Autodesk Fusion 360 part; units mm, degrees
sketch "Sketch1" plane through (0, 0, 0) normal (0, 1, 0) x (1, 0, 0)
  line L0 (37.303, -16.4637) -> (7.303, -16.4637)
  line L1 (-2.697, -16.4637) -> (-2.697, -12.4637)
  line L2 (2.303, -12.4637) -> (37.303, -12.4637)
  line L3 (37.303, -12.4637) -> (37.303, -16.4637)
  line L4 (37.303, -18.5137) -> (-5.6588, -18.5137) construction
  line L5 (2.303, -24.5637) -> (37.303, -24.5637)
  line L6 (-2.697, -20.5637) -> (-2.697, -24.5637)
  line L7 (37.303, -20.5637) -> (7.303, -20.5637)
  line L8 (37.303, -24.5637) -> (37.303, -20.5637)
  line L9 (-2.697, -16.4637) -> (-2.697, -20.5637)
  line L10 (7.303, -16.4637) -> (7.303, -20.5637)
  line L11 (2.303, -12.4637) -> (2.303, -2.4637)
  line L12 (2.303, -2.4637) -> (-2.697, -2.4637)
  line L13 (-2.697, -2.4637) -> (-2.697, -12.4637)
  line L14 (-2.697, -34.5637) -> (-2.697, -24.5637)
  line L15 (2.303, -34.5637) -> (-2.697, -34.5637)
  line L16 (2.303, -24.5637) -> (2.303, -34.5637)
  dimension "d4" = 4
  dimension "d5" = 10
  dimension "d6" = 5
  dimension "d7" = 10
extrude "Extrude1" add sketch "Sketch1" along normal blind 60
sketch "Sketch2" plane through (-2.697, 0, 0) normal (-1, 0, 0) x (0, -1, 0)
  line L0 (0, 2.4637) -> (0, 34.5637)
  line L1 (0, 34.5637) -> (-60, 34.5637)
  line L2 (-60, 34.5637) -> (-60, 2.4637)
  line L3 (-60, 2.4637) -> (0, 2.4637)
  circle A0 centre (-55, 7.4637) radius 1.75
  circle A1 centre (-48.4286, 7.4637) radius 1.75
  circle A2 centre (-41.8571, 7.4637) radius 1.75
  circle A3 centre (-35.2857, 7.4637) radius 1.75
  circle A4 centre (-28.7143, 7.4637) radius 1.75
  circle A5 centre (-22.1429, 7.4637) radius 1.75
  circle A6 centre (-15.5714, 7.4637) radius 1.75
  circle A7 centre (-9, 7.4637) radius 1.75
  circle A8 centre (-55, 30.4637) radius 1.75
  circle A9 centre (-48.4286, 30.4637) radius 1.75
  circle A10 centre (-41.8571, 30.4637) radius 1.75
  circle A11 centre (-35.2857, 30.4637) radius 1.75
  circle A12 centre (-28.7143, 30.4637) radius 1.75
  circle A13 centre (-22.1429, 30.4637) radius 1.75
  circle A14 centre (-15.5714, 30.4637) radius 1.75
  circle A15 centre (-9, 30.4637) radius 1.75
  dimension "d10" = 3.5
  dimension "d11" = 5
  dimension "d12" = 5
  dimension "d15" = 46
  dimension "d16" = 0
  dimension "d17" = 3.5
  dimension "d18" = 28
  dimension "d21" = 46
  dimension "d22" = 0
extrude "Extrude2" cut sketch "Sketch2" against normal blind 11 contours A0 | A1 | A2 | A3 | A4 | A5 | A6 | A7 | A8 | A9 | A10 | A11 | A12 | A13 | A14 | A15
For this review, take the finished solid that the model builds, in its own axes (mm). A direction names the side the tool comes from. Coordinates: 2 decimals unless noted, no trailing zeros. Write each loop counter-clockwise with the first axis right and the second up, starting at its lowest first coordinate (ties: lowest second). Pieces come first, ordered by that corner, then holes. Notation, with made-up numbers: (82.5, -36) - (109.5, -36) arc R15 ccw to (109.5, -21) - close; hole circle Ø6 at (84, -30). An arc over 180 degrees is marked (long way). Answer in a Markdown table with one row per item. Add a question column.
Q1. Draft analysis for pull direction Z (two halves, no side actions). For faces 4 (the flat face through (-2.697, 30, 19)), 5 (the flat face through (20, 30, 24.564)), 6 (the cylindrical face through (-0.232, 49.718, 31.646)), state which applies: +Z half, -Z half, draft (parallel to the pull), parting line (faces both ways), or undercut.
Q2. We need section B-B, the plane y = 55. State the section outline as (x, z) points, and give its area (3 significant figures).
Q3. For probe 1 along Z at (x, y) = (12.5, 49); probe 2 along Z at (x, y) = (-0.5, 29); probe 3 along X at (y, z) = (8, 4.5), list the stretches that pass through material, from the lowest coordinate up.
Q4. Tool access review of faces 1 (the flat face through (37.303, 30, 14)), 2 (the flat face through (23, 30, 20.564)), 3 (the flat face through (2.303, 30, 28)): name each direction out of +Z, -Z, +X, -X, +Y, -Y from which nothing blocks a thin tool from reaching the whole face with its end or side.
Q5. We need section C-C, the plane y = 19.5. State the section outline as (x, z) points.
Q6. We need section A-A, the plane x = 28. State the section outline as (y, z) points.
Q7. We need section D-D, the plane y = 29.5. State the section outline as (x, z) points.
Q8. For P1, Ø11, axis at y = 39, z = 31.5, coming from the +X side; P2, Ø3, axis at y = 15.57, z = 30.46, coming from the +X side; P3, Ø4.5, axis at y = 22, z = 19, coming from the +X side; P4, Ø10.5, axis at x = 22.5, y = 28, coming from the -Z side, all flat-tipped, find the tip position at first contact; note any pin that passes through.
Answer list:
| question | item | result |
|---|---|---|
| 1 | face 4 | draft |
| 1 | face 5 | +Z half |
| 1 | face 6 | undercut |
| 2 | outline | (-2.7, 2.46) - (2.3, 2.46) - (2.3, 5.71) - (-2.7, 5.71) - close; (-2.7, 9.21) - (2.3, 9.21) - (2.3, 12.46) - (37.3, 12.46) - (37.3, 16.46) - (7.3, 16.46) - (7.3, 20.56) - (37.3, 20.56) - (37.3, 24.56) - (2.3, 24.56) - (2.3, 28.71) - (-2.7, 28.71) - close; (-2.7, 32.21) - (2.3, 32.21) - (2.3, 34.56) - (-2.7, 34.56) - close |
| 2 | area | 426 mm2 |
| 3 | probe 1 | z = 12.46 to 16.46, 20.56 to 24.56 |
| 3 | probe 2 | z = 2.46 to 5.74, 9.19 to 28.74, 32.19 to 34.56 |
| 3 | probe 3 | x = -2.7 to 2.3 |
| 4 | face 1 | +Z, -Z, +X, +Y, -Y |
| 4 | face 2 | +X, +Y, -Y |
| 4 | face 3 | +Z, +X, +Y, -Y |
| 5 | outline | (-2.7, 2.46) - (2.3, 2.46) - (2.3, 12.46) - (37.3, 12.46) - (37.3, 16.46) - (7.3, 16.46) - (7.3, 20.56) - (37.3, 20.56) - (37.3, 24.56) - (2.3, 24.56) - (2.3, 34.56) - (-2.7, 34.56) - close |
| 6 | outline | (0, 12.46) - (60, 12.46) - (60, 16.46) - (0, 16.46) - close; (0, 20.56) - (60, 20.56) - (60, 24.56) - (0, 24.56) - close |
| 7 | outline | (-2.7, 2.46) - (2.3, 2.46) - (2.3, 5.9) - (-2.7, 5.9) - close; (-2.7, 9.03) - (2.3, 9.03) - (2.3, 12.46) - (37.3, 12.46) - (37.3, 16.46) - (7.3, 16.46) - (7.3, 20.56) - (37.3, 20.56) - (37.3, 24.56) - (2.3, 24.56) - (2.3, 28.9) - (-2.7, 28.9) - close; (-2.7, 32.03) - (2.3, 32.03) - (2.3, 34.56) - (-2.7, 34.56) - close |
| 8 | P1 | stops at x = 2.3 |
| 8 | P2 | passes through |
| 8 | P3 | stops at x = 37.3 |
| 8 | P4 | stops at z = 12.46 |
